Here's the drawing with two shaded views (mm, measured from the low corner). I have some questions. A direction names the side the tool comes from. Coordinates: 2 decimals unless noted, no trailing zeros. Write each loop counter-clockwise with the first axis right and the second up, starting at its lowest first coordinate (ties: lowest second). Pieces come first, ordered by that corner, then holes. Notation, with made-up numbers: (-1.75, -20.75) -> (43.25, -20.75) arc R31 ccw to (43.25, 14.25) -> close; hole circle Ø8 at (87, 36). An arc over 180 degrees is marked (long way). Put each result on its own line as item: value.
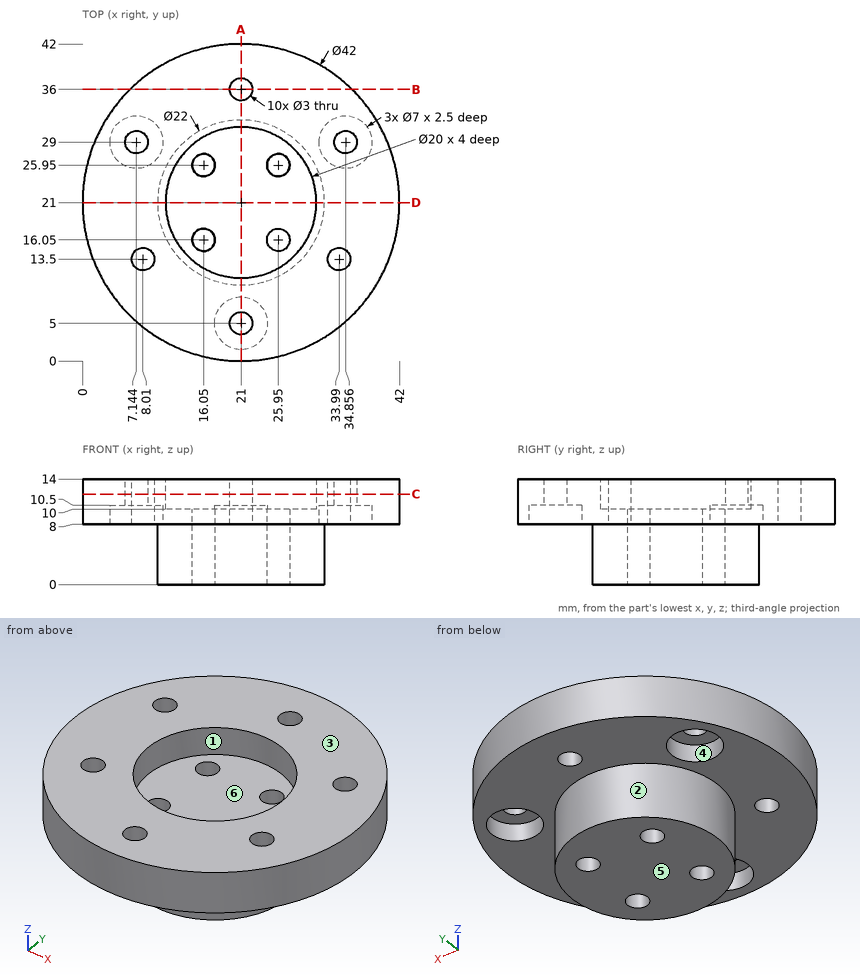
Item 1: Imagine slicing it at A-A on x = 21. Write out the boundary of the cut face in (y, z), then the cut area to 3 significant figures.
Output:
outline: (0, 8) -> (1.5, 8) -> (1.5, 10.5) -> (3.5, 10.5) -> (3.5, 14) -> (0, 14) -> close; (6.5, 10.5) -> (8.5, 10.5) -> (8.5, 8) -> (10, 8) -> (10, 0) -> (32, 0) -> (32, 8) -> (34.5, 8) -> (34.5, 14) -> (31, 14) -> (31, 10) -> (11, 10) -> (11, 14) -> (6.5, 14) -> close; (37.5, 8) -> (42, 8) -> (42, 14) -> (37.5, 14) -> close
area: 302 mm²
Item 2: For P1, Ø3.5, axis at x = 6.5, y = 29, coming from the -Z side; P2, Ø5, axis at x = 16.05, y = 25.95, coming from the -Z side; P3, Ø1.8, axis at x = 7.14, y = 29, coming from the -Z side; P4, Ø5, axis at x = 33.99, y = 13.5, coming from the -Z side, each with a flat end and sliding along its axis, tell me the tip position at first contact or that it passes through.
Output:
P1: stops at z = 10.5
P2: stops at z = 0
P3: passes through
P4: stops at z = 8
Item 3: Imagine slicing it at D-D on y = 21. Write out the boundary of the cut face in (x, z).
Output:
outline: (0, 8) -> (10, 8) -> (10, 0) -> (32, 0) -> (32, 8) -> (42, 8) -> (42, 14) -> (31, 14) -> (31, 10) -> (11, 10) -> (11, 14) -> (0, 14) -> close
Item 4: Imagine slicing it at C-C on z = 12. Write out the boundary of the cut face in (x, y).
Output:
outline: circle Ø42 at (21, 21); hole circle Ø3 at (7.14, 29); hole circle Ø3 at (8.01, 13.5); hole circle Ø20 at (21, 21); hole circle Ø3 at (21, 5); hole circle Ø3 at (21, 36); hole circle Ø3 at (33.99, 13.5); hole circle Ø3 at (34.86, 29)
Item 5: If we mould it in two halves opening along Y, with no side actions, what happens to the marked faces 1, 2 and 3? For each: released by +Y, released by -Y, zero draft, split by the parting line, or undercut.
Output:
face 1: undercut
face 2: split by the parting line
face 3: zero draft
Item 6: Which directions (+Z, -Z, +X, -X, +Y, -Y) give clear straight access to the entire face, cutting with the end or side of a thin tool? Please do the marked faces 4, 5 and 6.
Output:
face 4: -Z
face 5: -Z, +X, -X, +Y, -Y
face 6: +Z
Item 7: Please list where these lines run through material, in increasing order: line 1 along Y through (x, z) = (21, 10.8); line 2 along Y through (x, z) = (21, 9.45); line 3 along X through (y, z) = (14, 9.25) (1 decimal). Write a range as from..to.
Output:
line 1: y = 0..3.5, 6.5..11, 31..34.5, 37.5..42
line 2: y = 0..1.5, 8.5..34.5, 37.5..42
line 3: x = 1.2..6.6, 9.4..32.6, 35.4..40.8
Item 8: Imagine slicing it at B-B on y = 36. Write out the boundary of the cut face in (x, z).
Output:
outline: (6.3, 8) -> (19.5, 8) -> (19.5, 14) -> (6.3, 14) -> close; (22.5, 8) -> (35.7, 8) -> (35.7, 14) -> (22.5, 14) -> close
